The figure shows three views and two pictorial views of one solid part (mm, origin at its lowest corner). Answer the questions. A direction names the side the tool comes from. Coordinates: 2 decimals unless noted, no trailing zeros. Loops run counter-clockwise (first coordinate to the right, second up) from the corner with the lowest first, then second, coordinate; pieces in that order, holes last. Notation, with made-up numbers: M 69.25,-36.75 L 97.25,-36.75 A22 cw 97.25,-14.75 Z; hole C 32.25,66 d5. An arc over 180 degrees is marked long. Answer as a JSON object with one key per item and string values. Group by question number.
1. A cutting plane is placed at A-A on x = 1.9. Give the vertices of the cut face in (y, z).
2. A cutting plane is placed at C-C on z = 7.25. Give the vertices of the cut face in (x, y), and give its area (3 significant figures).
3. Given pin 1 (1 mm diameter, centred on x = 3, z = 5, fed in from -Y); pin 2 (1 mm diameter, centred on x = 3.5, y = 2, fed in from +Z); pin 3 (1.5 mm diameter, centred on y = 1.5, z = 4.5, fed in from +X), each flat-ended and moving along its own axis, determine where each tip first touches the part or whether it passes through.
4. For the marked faces 1 and 2, determine the directions among +Z, -Z, +X, -X, +Y, -Y from which every point of the face is accessible in a straight line to the end or side of a thin tool.
5. Straight lines are drawn through the part: L1, parallel to Z at x = 3.05, y = 1.4; L2, parallel to Y at x = 1.85, z = 4.75; L3, parallel to Y at x = 3.25, z = 1.5. For each, find the intervals that lie inside material, in ascending order.
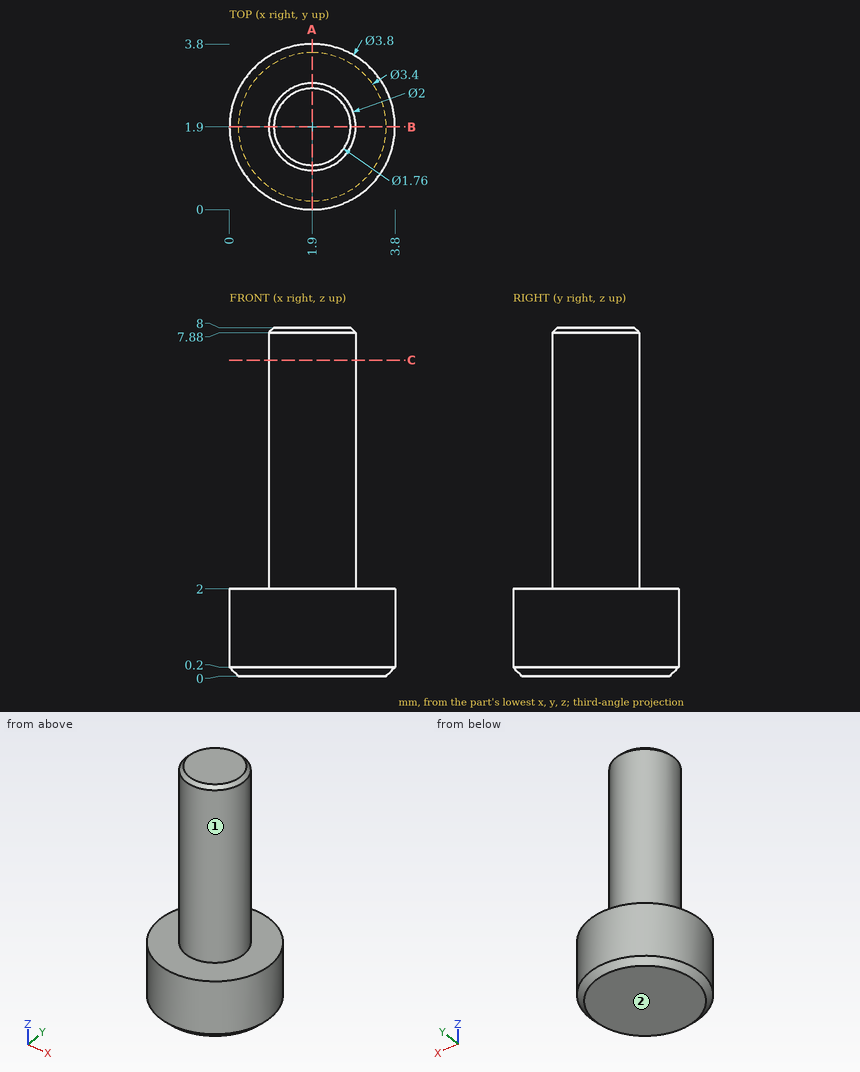
From the geometry:
{
 "1": {"outline": "M 0,0.2 L 0.2,0 L 3.6,0 L 3.8,0.2 L 3.8,2 L 2.9,2 L 2.9,7.88 L 2.78,8 L 1.02,8 L 0.9,7.88 L 0.9,2 L 0,2 Z"},
 "2": {"outline": "C 1.9,1.9 d2", "area": "3.14 mm²"},
 "3": {"pin 1": "stops at y = 1.1", "pin 2": "stops at z = 2", "pin 3": "stops at x = 2.9"},
 "4": {"face 1": "+Z", "face 2": "-Z, +X, -X, +Y, -Y"},
 "5": {"L1": "z = 0 to 2", "L2": "y = 0.9 to 2.9", "L3": "y = 0.56 to 3.24"}
}
